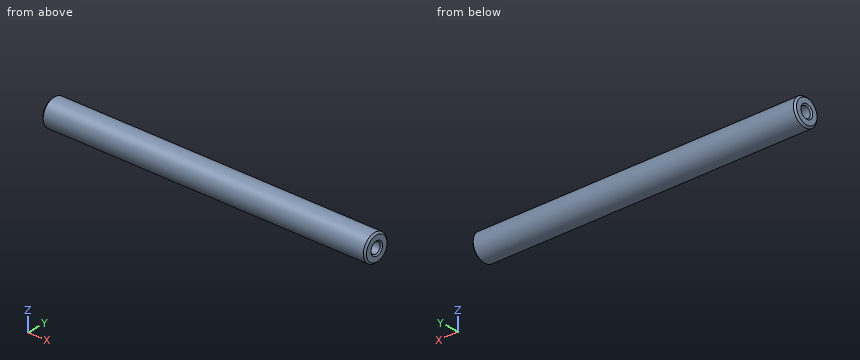
Autodesk Inventor part; units mm, degrees
ref_plane "YZ Plane" through (0, 0, 0) normal (1, 0, 0) x (0, 1, 0)
ref_plane "XZ Plane" through (0, 0, 0) normal (0, 1, 0) x (-1, 0, 0)
ref_plane "XY Plane" through (0, 0, 0) normal (0, 0, 1) x (1, 0, 0)
sketch "Sketch_1" plane through (0, 0, 0) normal (0, 0, 1) x (1, 0, 0)
  line L0 (98, 0) -> (0, 0)
  line L1 (0, 0) -> (0, 3.5)
  line L2 (0, 3.5) -> (0.5, 4)
  line L3 (0.5, 4) -> (97.5, 4)
  line L4 (97.5, 4) -> (98, 3.5)
  line L5 (98, 3.5) -> (98, 0)
  line L6 (98, 0) -> (0, 0)
revolve "Revolution1" add sketch "Sketch_1" angle 360 about axis through (98, 0, 0) along (1, 0, 0)
sketch "Sketch2" plane through (0, 0, 0) normal (-1, 0, 0) x (0, 0, 1)
  point P0 (0, 0)
hole "Hole1" at (0, 0, 0) direction (1, 0, 0) diameter 3.242 depth 13.0641 tip angle 120 countersink diameter 4 countersink angle 90
sketch "Sketch3" plane through (98, 0, 0) normal (1, 0, 0) x (0, 0, -1)
  point P0 (0, 0)
hole "Hole2" at (98, 0, 0) direction (-1, 0, 0) diameter 3.242 depth 13.0641 tip angle 120 countersink diameter 4 countersink angle 90
properties part number "SFHRW8-98-M4-N4" material "鋼、炭素鋼"
Here's how the part is built. I have some questions about the finished solid (model axes, mm). Give positions to 0.01 mm unless a question says otherwise; leave off trailing zeros. Loops run counter-clockwise (first coordinate to the right, second up) from the corner with the lowest first, then second, coordinate; pieces in that order, holes last. Notation, with made-up numbers: M 19.25,-39 L 25.25,-39 A26 cw 25.25,-15 Z; hole C 54.25,86 d3. An arc over 180 degrees is marked long. Use one line per item in the form item = value. Start each with the question number.
Q1. Will these pins go through, and if not, where does the flat tip stop? pin 1 Ø2.5 at (y, z) = (0, 0) entering from -X; pin 2 Ø1.5 at (x, y) = (84.5, 1) entering from +Z.
Q2. I need wall thicknesses on line 1 along Z through (x, y) = (94, 0); line 2 along Z through (x, y) = (19.5, -2); line 3 along Z through (x, y) = (76, -3.25). Which ranges of each line are inside material? Lowest first, please.
Q3. If we section it at A-A (x = 63): Write out the boundary of the cut face in (y, z).
Taken from the geometry:
q1.pin_1 = 13.28
q1.pin_2 = 3.99
q2.line_1 = -4 to -1.62, 1.62 to 4
q2.line_2 = -3.46 to 3.46
q2.line_3 = -2.33 to 2.33
q3.outline = C 0,0 d8
